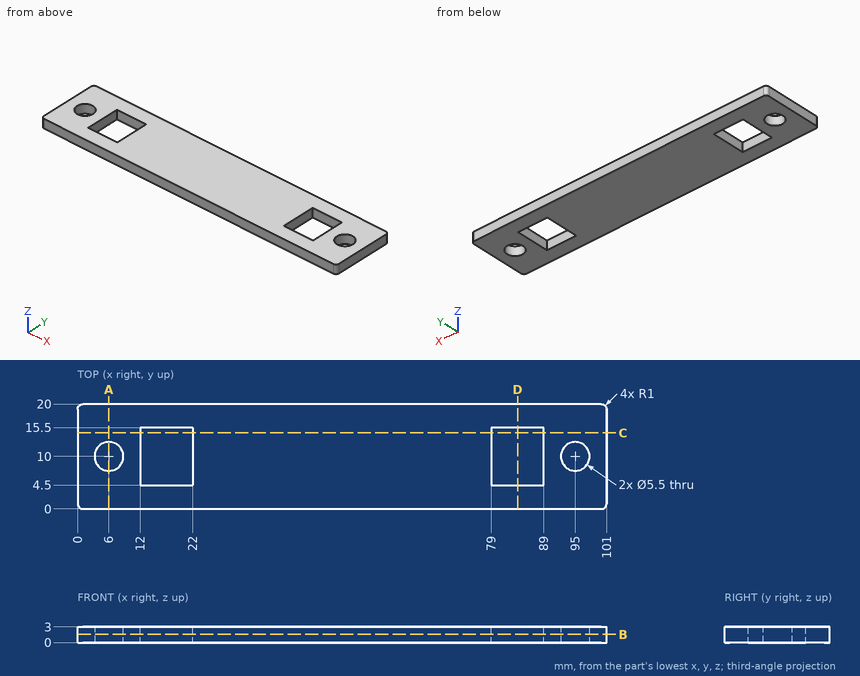
Can you work these out from the drawing? Everything is in mm from the part's minimum corner. Give positions to 0.01 mm unless a question says otherwise; leave off trailing zeros. Order: outer loops, then holes, each group sorted by start corner. A loop starts at its lowest first (then second) coordinate and runs counter-clockwise, first axis right, second up.
Item 1: If we section it at C-C, the plane y = 14.5: Write out the boundary of the cut face in (x, z).
Item 2: I'm going to push a flat-ended pin straight in: pin 1 (4.5 mm diameter, centred on x = 6, y = 10, fed in from -Z). Where does the tip first touch, or does it pass through?
Item 3: If we section it at B-B, the plane z = 1.55: Write out the boundary of the cut face in (x, y), plus the area to 3 significant figures.
Item 4: I need wall thicknesses on line 1 (X direction, y = 14.5, z = 1.2); line 2 (X direction, y = 10.25, z = 2.6); line 3 (Y direction, x = 6, z = 1.65). Which ranges of each line are inside material? Lowest first, please.
Item 5: If we section it at A-A, the plane x = 6: Write out the boundary of the cut face in (y, z), plus the area to 3 significant figures.
Item 6: If we section it at D-D, the plane x = 84: Write out the boundary of the cut face in (y, z).
Values:
1. outline: (0, 0) - (12, 0) - (12, 3) - (0, 3) - close; (22, 0) - (79, 0) - (79, 3) - (22, 3) - close; (89, 0) - (101, 0) - (101, 3) - (89, 3) - close
2. pin 1: passes through
3. outline: (0, 1) arc R1 ccw to (1, 0) - (100, 0) arc R1 ccw to (101, 1) - (101, 19) arc R1 ccw to (100, 20) - (1, 20) arc R1 ccw to (0, 19) - close; hole circle Ø5.5 at (6, 10); hole (12, 4.5) - (22, 4.5) - (22, 15.5) - (12, 15.5) - close; hole (79, 4.5) - (89, 4.5) - (89, 15.5) - (79, 15.5) - close; hole circle Ø5.5 at (95, 10)
3. area: 1,750 mm2
4. line 1: x = 0 to 12, 22 to 79, 89 to 101
4. line 2: x = 0 to 3.26, 8.74 to 12, 22 to 79, 89 to 92.26, 97.74 to 101
4. line 3: y = 0 to 7.25, 12.75 to 20
5. outline: (0, 0) - (7.25, 0) - (7.25, 3) - (0, 3) - close; (12.75, 0) - (20, 0) - (20, 3) - (12.75, 3) - close
5. area: 43.5 mm2
6. outline: (0, 0) - (4.5, 0) - (4.5, 3) - (0, 3) - close; (15.5, 0) - (20, 0) - (20, 3) - (15.5, 3) - close
